Check sheet for the modelled part. Datum: model origin and axes. Units: mm. Give positions to 0.01 mm unless a question says otherwise; leave off trailing zeros. Write each loop counter-clockwise with the first axis right and the second up, starting at its lowest first coordinate (ties: lowest second). Pieces come first, ordered by that corner, then holes. Notation, with made-up numbers: (83.5, -14) -> (122.5, -14) arc R31 ccw to (122.5, 16) -> close; hole circle Ø5 at (62.5, 51). An arc over 180 degrees is marked (long way). Write each question's results on one line, items separated by ' | '. Start each with the question number.
Autodesk Inventor part; units mm, degrees
ref_plane "YZ Plane" through (0, 0, 0) normal (1, 0, 0) x (0, 1, 0)
ref_plane "XZ Plane" through (0, 0, 0) normal (0, 1, 0) x (-1, 0, 0)
ref_plane "XY Plane" through (0, 0, 0) normal (0, 0, 1) x (1, 0, 0)
sketch "Sketch1" plane through (0, 0, 0) normal (0, 1, 0) x (-1, 0, 0)
  line L0 (-101.6, -127) -> (50.8, -127)
  line L1 (50.8, -127) -> (50.8, 127)
  line L2 (50.8, 127) -> (-101.6, 127)
  line L3 (-101.6, 127) -> (-101.6, -127)
  point P0 (0, 0)
  dimension "d0" = 152.4
  dimension "d1" = 254
extrude "Extrusion2" add sketch "Sketch1" along normal blind 1.5875
sketch "Sketch3" plane through (0, 1.5875, 0) normal (0, 1, 0) x (1, 0, 0)
  circle A0 centre (63.5, -114.3) radius 2.1844
  circle A1 centre (-12.7, -114.3) radius 2.1844
  point P0 (0, 0)
  dimension "d13" = 4.3688
  dimension "d14" = 4.3688
hole "Hole1" at (63.5, 1.5875, 114.3) at (-12.7, 1.5875, 114.3) direction (0, -1, 0) diameter 4.3688 end through all
sketch "Sketch4" plane through (0, 0, 0) normal (0, -1, 0) x (1, 0, 0)
  line L0 (101.6, 127) -> (101.6, -127)
  line L1 (-50.8, -127) -> (-50.8, 127)
  line L2 (101.6, 50.8) -> (254, 50.8) construction
  line L3 (-12.7, 34.925) -> (-12.7, 66.675)
  line L4 (63.5, 66.675) -> (63.5, 34.925)
  line L5 (-12.7, 66.675) -> (-12.7, 69.85)
  line L6 (63.5, 73.025) -> (-12.7, 73.025)
  line L7 (-12.7, 73.025) -> (-12.7, 28.575)
  line L8 (-12.7, 28.575) -> (63.5, 28.575)
  line L9 (63.5, 28.575) -> (63.5, 73.025)
  point P0 (0, 0)
  point P1 (-12.7, 31.75)
  point P2 (63.5, 69.85)
  dimension "d24" = 76.2
  dimension "d25" = 38.1
extrude "Extrusion5" cut sketch "Sketch4" against normal up to next
properties part number "2polycarb10x6" material "Polycarbonate, Clear"
Item 1: Section check B-B on y = 1.2. Record the boundary of the cut face in (x, z) (3 decimals), then the cut area to 3 significant figures.
Item 2: Depth check by flat-ended pin: pin 1 Ø5 at (x, z) = (85, -15.5) entering from -Y; pin 2 Ø4 at (x, z) = (-12.7, 114.3) entering from -Y. Enter the tip coordinate at first touch or a pass-through.
Item 3: Thickness scan on probe 1 along X at (y, z) = (0.6, 114.3); probe 2 along Z at (x, y) = (21.5, 0.75) (3 decimals); probe 3 along Z at (x, y) = (64, 1.3). Record the ranges inside material, lowest first. Write a range as from..to.
Item 4: Section check A-A on x = 6.5. Record the boundary of the cut face in (y, z) (1 decimal).
Check sheet entries:
1) outline: (-50.8, -127) -> (101.6, -127) -> (101.6, 127) -> (-50.8, 127) -> close; hole circle Ø4.369 at (-12.7, 114.3); hole (-12.7, 28.575) -> (63.5, 28.575) -> (63.5, 73.025) -> (-12.7, 73.025) -> close; hole circle Ø4.369 at (63.5, 114.3) | area: 35,300 mm^2
2) pin 1: stops at y = 0 | pin 2: passes through
3) probe 1: x = -50.8..-14.88, -10.52..61.32, 65.68..101.6 | probe 2: z = -127..28.575, 73.025..127 | probe 3: z = -127..112.17, 116.43..127
4) outline: (0, -127) -> (1.6, -127) -> (1.6, 28.6) -> (0, 28.6) -> close; (0, 73) -> (1.6, 73) -> (1.6, 127) -> (0, 127) -> close
